Check sheet for the modelled part. Datum: model origin and axes. Units: mm. Round coordinates to 2 decimals unless told otherwise and drop trailing zeros. Write each loop counter-clockwise with the first axis right and the second up, starting at its lowest first coordinate (ties: lowest second). Pieces come first, ordered by that corner, then holes. Notation, with made-up numbers: (55, 53) - (78, 53) arc R17 ccw to (78, 60) - close; hole circle Ø10 at (61.25, 29.5). An arc over 180 degrees is marked (long way). Answer as a JSON object with one key per item and string values. Group by question number.
Item 1: Sectioned sample at A-A on y = 2.3. Count the separate pieces of the cut face and the enclosed holes in it, plus the area to 3 significant figures.
Item 2: Thickness scan on line 1 (X direction, y = 2.15, z = -28); line 2 (Z direction, x = 2, y = 2.2); line 3 (X direction, y = 1.9, z = 9). Record the ranges inside material, lowest first.
Item 3: Sectioned sample at B-B on z = 0. Record the boundary of the cut face in (x, y), plus the area to 3 significant figures.
Item 4: Sectioned sample at C-C on z = -18.5. Record the boundary of the cut face in (x, y).
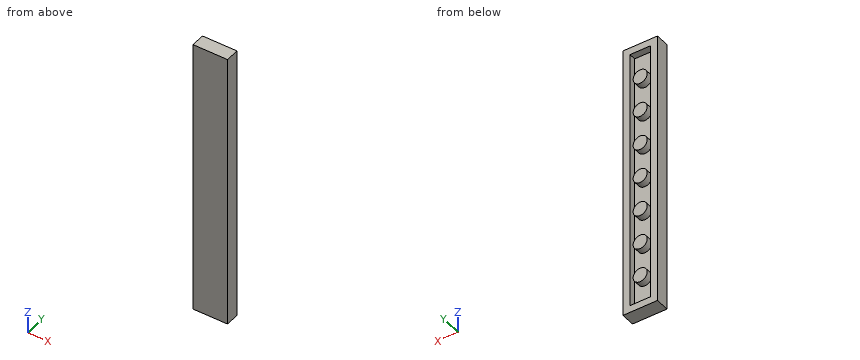
```python
from build123d import *

# Parameters (mm, degrees)
SKETCH1_W           = 8.065
SKETCH1_H           = 64.52
BOSS_EXTRUDE1_DEPTH = 3.226
CUT_EXTRUDE1_DEPTH  = 1.5835
SKETCH7_W           = 1.6425
SKETCH7_H           = 1.5835
SKETCH8_W           = 1.6425
SKETCH8_H           = 1.5835
SKETCH9_W           = 1.6425
SKETCH9_H           = 1.5835
LPATTERN1_COUNT     = 5
LPATTERN1_PITCH     = 8.065


with BuildPart() as part:
    # Sketch1 → Boss-Extrude1 (new body)
    with BuildSketch(Plane(origin=(0, 3.226, 0), x_dir=(1, 0, 0), z_dir=(0, 1, 0))):
        with Locations((0, 16.13)):
            Rectangle(SKETCH1_W, SKETCH1_H)
    extrude(amount=-BOSS_EXTRUDE1_DEPTH)

    # Sketch2 → Cut-Extrude1 (cut)
    with BuildSketch(Plane(origin=(0, 3.226, 0), x_dir=(-1, 0, 0), z_dir=(0, 1, 0))):
        Polygon((2.39, 14.4875), (-2.39, 14.4875), (-2.39, -14.4875), (-2.39, -46.7475), (2.39, -46.7475), (2.39, -14.4875), align=None)
    extrude(amount=-CUT_EXTRUDE1_DEPTH, mode=Mode.SUBTRACT)

    # Sketch7 → Revolve5 (revolve)
    with BuildSketch(Plane(origin=(0, 0, -8.065), x_dir=(-1, 0, 0), z_dir=(0, 0, -1)), mode=Mode.PRIVATE) as revolve5_sk:
        with Locations((-0.82125, 2.43425)):
            Rectangle(SKETCH7_W, SKETCH7_H)
    revolve5 = revolve(revolve5_sk.sketch.rotate(Axis((0, 1.6425, -8.065), (0, 1, 0)), 270), axis=Axis((0, 1.6425, -8.065), (0, 1, 0)))

    # Sketch8 → Revolve6 (revolve)
    with BuildSketch(Plane(origin=(0, 0, 0), x_dir=(-1, 0, 0), z_dir=(0, 0, -1)), mode=Mode.PRIVATE) as revolve6_sk:
        with Locations((-0.82125, 2.43425)):
            Rectangle(SKETCH8_W, SKETCH8_H)
    revolve(revolve6_sk.sketch.rotate(Axis((0, 1.6425, 0), (0, 1, 0)), 270), axis=Axis((0, 1.6425, 0), (0, 1, 0)))

    # Sketch9 → Revolve7 (revolve)
    with BuildSketch(Plane(origin=(0, 0, 8.065), x_dir=(-1, 0, 0), z_dir=(0, 0, -1)), mode=Mode.PRIVATE) as revolve7_sk:
        with Locations((-0.82125, 2.43425)):
            Rectangle(SKETCH9_W, SKETCH9_H)
    revolve(revolve7_sk.sketch.rotate(Axis((0, 1.6425, 8.065), (0, 1, 0)), 270), axis=Axis((0, 1.6425, 8.065), (0, 1, 0)))

    # LPattern1: Revolve5 ×5
    with Locations(*[(0, 0, -i * LPATTERN1_PITCH) for i in range(1, LPATTERN1_COUNT)]):
        add(revolve5)


solid = part.part
```
Completed:
{
 "1": {"separate pieces": "8", "enclosed holes": "1", "area": "287 mm²"},
 "2": {"line 1": "-4.03 to -2.39, 2.39 to 4.03", "line 2": "-48.39 to -46.75, 14.49 to 16.13", "line 3": "-4.03 to -2.39, -1.35 to 1.35, 2.39 to 4.03"},
 "3": {"outline": "(-4.03, 0) - (4.03, 0) - (4.03, 3.23) - (2.39, 3.23) - (2.39, 1.64) - (1.64, 1.64) - (1.64, 3.23) - (-1.64, 3.23) - (-1.64, 1.64) - (-2.39, 1.64) - (-2.39, 3.23) - (-4.03, 3.23) - close", "area": "23.7 mm²"},
 "4": {"outline": "(-4.03, 0) - (4.03, 0) - (4.03, 3.23) - (2.39, 3.23) - (2.39, 1.64) - (-2.39, 1.64) - (-2.39, 3.23) - (-4.03, 3.23) - close"}
}
